from build123d import *

# Parameters (mm, degrees)
F0_W      = 104.96
F0_H      = 107.52
F0_W_2    = 6.23
F0_H_2    = 6.61
F0_R      = 1
F1_DEPTH  = 3.5
F2_DEPTH  = 22
F3_T      = -2.5
F4_DEPTH  = 3.501
F5_DEPTH  = 5
F5_FACE_R = 1
F6_DEPTH  = 1
F7_DEPTH  = 5
F8_DEPTH  = 5
F9_R      = 1.35
F10_DEPTH = 19.05


with BuildPart() as f1:
    # F0 (on Top) → F1 (new body)
    with BuildSketch(Plane.XY):
        with Locations((0, -17.5)):
            Rectangle(F0_W, F0_H)
        Polygon((-48.71, 28.26), (-42.48, 28.26), (42.48, 28.26), (48.71, 28.26), (48.71, 21.65), (42.48, 21.65), (42.48, -21.65), (48.71, -21.65), (48.71, -28.26), (42.48, -28.26), (-42.48, -28.26), (-48.71, -28.26), (-48.71, -21.65), (-42.48, -21.65), (-42.48, 21.65), (-48.71, 21.65), align=None, mode=Mode.SUBTRACT)
        with Locations((-45.595, -24.955)):
            Rectangle(F0_W_2, F0_H_2)
        with Locations((-45.595, -24.955)):
            Circle(F0_R, mode=Mode.SUBTRACT)
        with Locations((-45.595, 24.955)):
            Rectangle(F0_W_2, F0_H_2)
        with Locations((-45.595, 24.955)):
            Circle(F0_R, mode=Mode.SUBTRACT)
        with Locations((-45.595, 24.955)):
            Circle(F0_R)
        with Locations((-45.595, -24.955)):
            Circle(F0_R)
        with Locations((45.595, -24.955)):
            Rectangle(F0_W_2, F0_H_2)
        with Locations((45.595, -24.955)):
            Circle(F0_R, mode=Mode.SUBTRACT)
        with Locations((45.595, -24.955)):
            Circle(F0_R)
        with Locations((45.595, 24.955)):
            Rectangle(F0_W_2, F0_H_2)
        with Locations((45.595, 24.955)):
            Circle(F0_R, mode=Mode.SUBTRACT)
        with Locations((45.595, 24.955)):
            Circle(F0_R)
        Polygon((42.48, 28.26), (-42.48, 28.26), (-42.48, 21.65), (-42.48, -21.65), (-42.48, -28.26), (42.48, -28.26), (42.48, -21.65), (42.48, 21.65), align=None)
    extrude(amount=-F1_DEPTH)

    # F0 (on Top) → F2 (join)
    with BuildSketch(Plane.XY):
        with Locations((0, -17.5)):
            Rectangle(F0_W, F0_H)
        Polygon((-48.71, 28.26), (-42.48, 28.26), (42.48, 28.26), (48.71, 28.26), (48.71, 21.65), (42.48, 21.65), (42.48, -21.65), (48.71, -21.65), (48.71, -28.26), (42.48, -28.26), (-42.48, -28.26), (-48.71, -28.26), (-48.71, -21.65), (-42.48, -21.65), (-42.48, 21.65), (-48.71, 21.65), align=None, mode=Mode.SUBTRACT)
        with Locations((-45.595, -24.955)):
            Rectangle(F0_W_2, F0_H_2)
        with Locations((-45.595, -24.955)):
            Circle(F0_R, mode=Mode.SUBTRACT)
        with Locations((-45.595, 24.955)):
            Rectangle(F0_W_2, F0_H_2)
        with Locations((-45.595, 24.955)):
            Circle(F0_R, mode=Mode.SUBTRACT)
        with Locations((45.595, 24.955)):
            Rectangle(F0_W_2, F0_H_2)
        with Locations((45.595, 24.955)):
            Circle(F0_R, mode=Mode.SUBTRACT)
        with Locations((45.595, -24.955)):
            Rectangle(F0_W_2, F0_H_2)
        with Locations((45.595, -24.955)):
            Circle(F0_R, mode=Mode.SUBTRACT)
        with Locations((-45.595, -24.955)):
            Circle(F0_R)
        with Locations((-45.595, 24.955)):
            Circle(F0_R)
        with Locations((45.595, 24.955)):
            Circle(F0_R)
        with Locations((45.595, -24.955)):
            Circle(F0_R)
        Polygon((42.48, 28.26), (-42.48, 28.26), (-42.48, 21.65), (-42.48, -21.65), (-42.48, -28.26), (42.48, -28.26), (42.48, -21.65), (42.48, 21.65), align=None)
    extrude(amount=F2_DEPTH)

    # F3
    f3_openings = [f1.faces().sort_by_distance(p)[0] for p in [
        (0, -17.5, 22),
    ]]
    offset(amount=F3_T, openings=f3_openings)

    # F0 (on Top) → F4 (cut, through all)
    with BuildSketch(Plane.XY):
        Polygon((42.48, 28.26), (-42.48, 28.26), (-42.48, 21.65), (-42.48, -21.65), (-42.48, -28.26), (42.48, -28.26), (42.48, -21.65), (42.48, 21.65), align=None)
    extrude(amount=-F4_DEPTH, mode=Mode.SUBTRACT)



with BuildPart() as f5:
    # F0 (on Top) → F5 (new body)
    with BuildSketch(Plane.XY):
        with Locations((-45.595, -24.955)):
            Circle(F0_R)
    extrude(amount=F5_DEPTH)


with BuildPart() as f5b:
    # F0 (on Top) → F5, piece 2 (new body)
    with BuildSketch(Plane.XY):
        with Locations((45.595, 24.955)):
            Circle(F0_R)
    extrude(amount=F5_DEPTH)


with BuildPart() as f5c:
    # F0 (on Top) → F5, piece 3 (new body)
    with BuildSketch(Plane.XY):
        with Locations((45.595, -24.955)):
            Circle(F0_R)
    extrude(amount=F5_DEPTH)


with BuildPart() as f5d:
    # F0 (on Top) → F5, piece 4 (new body)
    with BuildSketch(Plane.XY):
        with Locations((-45.595, 24.955)):
            Circle(F0_R)
    extrude(amount=F5_DEPTH)


with BuildPart() as f1_1:
    add(f1.part)

    add(f5.part)  # F6 merges F5

    add(f5b.part)  # F6 merges F5b

    add(f5c.part)  # F6 merges F5c

    add(f5d.part)  # F6 merges F5d
    # F5_face (on face) → F6 (join)
    with BuildSketch(Plane(origin=(-45.595, 24.955, 0), x_dir=(1, 0, 0), z_dir=(0, 0, -1))):
        Circle(F5_FACE_R)
        with Locations((0, 49.91)):
            Circle(F5_FACE_R)
        with Locations((91.19, 49.91)):
            Circle(F5_FACE_R)
        with Locations((91.19, 0)):
            Circle(F5_FACE_R)
    extrude(amount=F6_DEPTH)

    # F7 (add): a face of the model
    f7_faces = [f1_1.faces().sort_by_distance(p)[0] for p in [
        (0, 33.76, 10.5),
    ]]
    extrude(f7_faces, amount=F7_DEPTH)

    # F8 (add): a face of the model
    f8_faces = [f1_1.faces().sort_by_distance(p)[0] for p in [
        (0, -68.76, 10.5),
    ]]
    extrude(f8_faces, amount=F8_DEPTH)

    # F9 (on face) → F10 (cut)
    with BuildSketch(Plane.XY.offset(22)):
        with Locations((-48.73, 32.51)):
            Circle(F9_R)
        with Locations((48.73, 32.51)):
            Circle(F9_R)
        with Locations((-48.73, -67.51)):
            Circle(F9_R)
        with Locations((48.73, -67.51)):
            Circle(F9_R)
    extrude(amount=-F10_DEPTH, mode=Mode.SUBTRACT)


solid = f1_1.part
Can you work these out from the model? Positions are in its coordinate system, mm. A direction names the side the tool comes from. Round coordinates to 2 decimals unless told otherwise and drop trailing zeros. Loops run counter-clockwise (first coordinate to the right, second up) from the corner with the lowest first, then second, coordinate; pieces in that order, holes last. Notation, with made-up numbers: (48, 43) - (93, 43) arc R18 cw to (93, 75) - close; hole circle Ø4 at (-6.75, -34). An arc over 180 degrees is marked (long way). Answer in a Markdown table with one row per item. Add a question column.
Q1. For pin 1 Ø10 at (x, y) = (34, -31) entering from +Z; pin 2 Ø1.3 at (x, y) = (-49, -67) entering from +Z; pin 3 Ø1 at (x, y) = (45.5, 24.5) entering from +Z, each with a flat end and sliding along its axis, tell me the tip position at first contact or that it passes through.
Q2. Which directions (+Z, -Z, +X, -X, +Y, -Y) give clear straight access to the entire face, cutting with the end or side of a thin tool? Please do faces 4 (the cylindrical face through (-47.442, 32.916, 12.608)), 5 (the flat face through (-52.48, -18, 9)), 6 (the flat face through (-1, -28.26, -2)).
Q3. I want a section at A-A on y = 17.5. List the corners of the cut face in (x, z) for me, and give its area (3 significant figures).
Q4. I want a section at D-D on y = -43.5. List the corners of the cut face in (x, z) for me.
Q5. I need wall thicknesses on L1, parallel to X at y = -67.51, z = 9.25; L2, parallel to Y at x = 48.73, z = 13.25; L3, parallel to Y at x = -16.5, z = 17.75. Which ranges of each line are inside material? Lowest first, please.
Q6. We'd pull the mould along Y, two halves only. Please class faces 1 (the flat face through (-49, -67, 2.95)), 2 (the flat face through (52.48, -18, 9)), 3 (the flat face through (-1, -71.26, 9)): pulls with the +Y half, pulls with the -Y half, needs draft (parallel to the pull), parting line crosses it, or undercut.
Q7. I want a section at B-B on z = 18.25. List the corners of the cut face in (x, y) for me.
Q8. I want a section at C-C on x = -26.5. List the corners of the cut face in (y, z) for me.
A:
| question | item | result |
|---|---|---|
| 1 | pin 1 | z = -1 |
| 1 | pin 2 | z = 2.95 |
| 1 | pin 3 | z = 5 |
| 2 | face 4 | +Z |
| 2 | face 5 | +Z, -Z, -X, +Y, -Y |
| 2 | face 6 | +Z, -Z |
| 3 | outline | (-52.48, -3.5) - (-42.48, -3.5) - (-42.48, -1) - (-49.98, -1) - (-49.98, 22) - (-52.48, 22) - close; (42.48, -3.5) - (52.48, -3.5) - (52.48, 22) - (49.98, 22) - (49.98, -1) - (42.48, -1) - close |
| 3 | area | 165 mm^2 |
| 4 | outline | (-52.48, -3.5) - (52.48, -3.5) - (52.48, 22) - (49.98, 22) - (49.98, -1) - (-49.98, -1) - (-49.98, 22) - (-52.48, 22) - close |
| 5 | L1 | -52.48 to -50.08, -47.38 to 47.38, 50.08 to 52.48 |
| 5 | L2 | -71.26 to -68.86, -66.16 to -63.76, 28.76 to 31.16, 33.86 to 36.26 |
| 5 | L3 | -71.26 to -63.76, 28.76 to 36.26 |
| 6 | face 1 | undercut |
| 6 | face 2 | needs draft |
| 6 | face 3 | pulls with the -Y half |
| 7 | outline | (-52.48, -71.26) - (52.48, -71.26) - (52.48, 36.26) - (-52.48, 36.26) - close; hole circle Ø2.7 at (-48.73, -67.51); hole circle Ø2.7 at (-48.73, 32.51); hole (-49.98, -63.76) - (49.98, -63.76) - (49.98, 28.76) - (-49.98, 28.76) - close; hole circle Ø2.7 at (48.73, -67.51); hole circle Ø2.7 at (48.73, 32.51) |
| 8 | outline | (-71.26, -3.5) - (-28.26, -3.5) - (-28.26, -1) - (-63.76, -1) - (-63.76, 22) - (-71.26, 22) - close; (28.26, -3.5) - (36.26, -3.5) - (36.26, 22) - (28.76, 22) - (28.76, -1) - (28.26, -1) - close |
